Can you work these out from the model? Positions are in its coordinate system, mm. A direction names the side the tool comes from. Give positions to 0.01 mm unless a question says otherwise; leave off trailing zeros. Loops run counter-clockwise (first coordinate to the right, second up) from the corner with the lowest first, then second, coordinate; pieces in that order, holes last.
from build123d import *

# Parameters (mm, degrees)
F0_W     = 45
F0_H     = 75
F1_DEPTH = 30
F2_W     = 39
F2_H     = 69
F3_DEPTH = 27
F4_R     = 5
F5_R     = 1
F6_DEPTH = 3


with BuildPart() as f1:
    # F0 (on Top) → F1 (new body)
    with BuildSketch(Plane.XY):
        Rectangle(F0_W, F0_H)
    extrude(amount=F1_DEPTH)

    # F2 (on face) → F3 (cut)
    with BuildSketch(Plane.XY.offset(30)):
        Rectangle(F2_W, F2_H)
    extrude(amount=-F3_DEPTH, mode=Mode.SUBTRACT)

    # F4
    f4_edges = [f1.edges().sort_by_distance(p)[0] for p in [
        (22.5, -37.5, 15),
        (-22.5, -37.5, 15),
        (22.5, 37.5, 15),
        (-22.5, 37.5, 15),
    ]]
    fillet(f4_edges, radius=F4_R)

    # F5 (on face) → F6 (cut)
    with BuildSketch(Plane.YZ.offset(22.5)):
        with Locations((0, 25)):
            Circle(F5_R)
    extrude(amount=-F6_DEPTH, mode=Mode.SUBTRACT)


solid = f1.part
(1) Will this pin go through, and if not, where does the flat tip stop? P1, Ø5, axis at x = 5, y = 14, coming from the +Z side.
Returned:
P1: stops at z = 3
(2) Thinking about a two-plate mould opening in X: for faces 4 (the flat face through (-22.5, 0, 15)), 5 (the flat face through (-20, 0, 30)), 6 (the flat face through (-19.5, 0, 17)), 7 (the flat face through (0, -34.5, 17)), which applies, pulls with the +X half, pulls with the -X half, needs draft (parallel to the pull), parting line crosses it, or undercut?
Returned:
face 4: pulls with the -X half
face 5: needs draft
face 6: undercut
face 7: undercut
(3) Please list where these lines run through material, in increasing order: probe 1 along X at (y, z) = (-14, 15.75); probe 2 along Y at (x, z) = (-13.5, 3.5); probe 3 along Z at (x, y) = (20.9, 0).
Returned:
probe 1: x = -22.5 to -19.5, 19.5 to 22.5
probe 2: y = -37.5 to -34.5, 34.5 to 37.5
probe 3: z = 0 to 24, 26 to 30
(4) Suppose I cut it at B-B on z = 28. List the corners of the cut face in (x, y) for me.
Returned:
outline: (-22.5, -32.5) arc R5 ccw to (-17.5, -37.5) - (17.5, -37.5) arc R5 ccw to (22.5, -32.5) - (22.5, 32.5) arc R5 ccw to (17.5, 37.5) - (-17.5, 37.5) arc R5 ccw to (-22.5, 32.5) - close; hole (-19.5, -34.5) - (19.5, -34.5) - (19.5, 34.5) - (-19.5, 34.5) - close
(5) Which directions (+Z, -Z, +X, -X, +Y, -Y) give clear straight access to the entire face, cutting with the end or side of a thin tool? Please do faces 1 (the cylindrical face through (21, 0, 24)), 2 (the cylindrical face through (21, -36.07, 15.21)), 3 (the flat face through (0, 0, 3)).
Returned:
face 1: +X
face 2: +Z, -Z, +X, -Y
face 3: +Z
(6) Suppose I cut it at A-A on y = 0. List the corners of the cut face in (x, z) for me, plus the area to 3 significant figures.
Returned:
outline: (-22.5, 0) - (22.5, 0) - (22.5, 24) - (19.5, 24) - (19.5, 3) - (-19.5, 3) - (-19.5, 30) - (-22.5, 30) - close; (19.5, 26) - (22.5, 26) - (22.5, 30) - (19.5, 30) - close
area: 291 mm2
(7) Suppose I cut it at C-C on x = -6. List the corners of the cut face in (y, z) for me, plus the area to 3 significant figures.
Returned:
outline: (-37.5, 0) - (37.5, 0) - (37.5, 30) - (34.5, 30) - (34.5, 3) - (-34.5, 3) - (-34.5, 30) - (-37.5, 30) - close
area: 387 mm2
(8) Suppose I cut it at D-D on y = 30.5. List the corners of the cut face in (x, z) for me.
Returned:
outline: (-22.5, 0) - (22.5, 0) - (22.5, 30) - (19.5, 30) - (19.5, 3) - (-19.5, 3) - (-19.5, 30) - (-22.5, 30) - close
